Read the model definition and answer for the solid it produces. Units are mm, in the model's axes. A direction names the side the tool comes from. Give positions to 0.01 mm unless a question says otherwise; leave off trailing zeros. Write each loop counter-clockwise with the first axis right and the second up, starting at its lowest first coordinate (ties: lowest second). Pieces come first, ordered by that corner, then holes. Notation, with made-up numbers: M 10.5,31 L 48.5,31 A25 cw 48.5,60 Z; hole C 48.25,78 d6. An arc over 180 degrees is marked long. Put each result on its own line as item: value.
from build123d import *

# Parameters (mm, degrees)
SKETCH1_W           = 40
SKETCH1_H           = 12
SKETCH1_R           = 2
BOSS_EXTRUDE1_DEPTH = 5
SKETCH2_W           = 30.175
SKETCH2_H           = 10
BOSS_EXTRUDE2_DEPTH = 6
SKETCH3_R           = 3.175
CUT_EXTRUDE1_DEPTH  = 17


with BuildPart() as part:
    # Sketch1 → Boss-Extrude1 (new body)
    with BuildSketch(Plane(origin=(0, 0, 0), x_dir=(0, 0, -1), z_dir=(1, 0, 0))):
        Rectangle(SKETCH1_W, SKETCH1_H)
        with Locations((-16, 0)):
            Circle(SKETCH1_R, mode=Mode.SUBTRACT)
        with Locations(Location((16, 0, 0), (0, 0, 180))):
            Circle(SKETCH1_R, mode=Mode.SUBTRACT)
    extrude(amount=BOSS_EXTRUDE1_DEPTH)

    # Sketch2 → Boss-Extrude2 (add, symmetric)
    with BuildSketch(Plane(origin=(0, 0, 0), x_dir=(1, 0, 0), z_dir=(0, 1, 0))):
        with Locations((20.0875, 0)):
            Rectangle(SKETCH2_W, SKETCH2_H)
    extrude(amount=BOSS_EXTRUDE2_DEPTH, both=True)

    # Sketch3 → Cut-Extrude1 (cut, symmetric)
    with BuildSketch(Plane.XY):
        with Locations((35.18, 0)):
            Circle(SKETCH3_R)
    extrude(amount=CUT_EXTRUDE1_DEPTH, both=True, mode=Mode.SUBTRACT)


solid = part.part
(1) Section D-D on z = 8 is taken. Determine the outline of the cut face in (x, y).
Result:
outline: M 0,-6 L 5,-6 L 5,6 L 0,6 Z
(2) Which of the six approach directions +Z, -Z, +X, -X, +Y, -Y give full straight-line access (tool end or side, diameter ignored) to faces 1 (the face through (5, 0, -12)), 2 (the face through (0, 0, 0)), 3 (the face through (5, 0, 13))?
Result:
face 1: -Z, +X, +Y, -Y
face 2: +Z, -Z, -X, +Y, -Y
face 3: +Z, +X, +Y, -Y
(3) Section A-A on y = 0 is taken. Determine the outline of the cut face in (x, z) (3 decimals), and give its area (3 significant figures).
Result:
outline: M 0,-20 L 5,-20 L 5,-18 L 0,-18 Z; M 0,-14 L 5,-14 L 5,-5 L 32.005,-5 L 32.005,5 L 5,5 L 5,14 L 0,14 Z; M 0,18 L 5,18 L 5,20 L 0,20 Z
area: 430 mm²
(4) For a pull along Y with two mould halves and no side action, classify faces 4 (the face through (20, 0, -5)), 5 (the face through (13, -6, 0)), 6 (the face through (32.006, 0.07, 0.07)) as +Y half, -Y half, draft (parallel to the pull), parting line (faces both ways), or undercut.
Result:
face 4: draft
face 5: -Y half
face 6: undercut
(5) Section B-B on z = 16 is taken. Determine the outline of the cut face in (x, y), and give its area (3 significant figures).
Result:
outline: M 0,-6 L 5,-6 L 5,-2 L 0,-2 Z; M 0,2 L 5,2 L 5,6 L 0,6 Z
area: 40.0 mm²
(6) Section C-C on y = -4.25 is taken. Determine the outline of the cut face in (x, z) (3 decimals).
Result:
outline: M 0,-20 L 5,-20 L 5,-5 L 35.175,-5 L 35.175,5 L 5,5 L 5,20 L 0,20 Z
(7) Straight lines are drawn through the part: line 1 along Y through (x, z) = (1, -16); line 2 along Z through (x, y) = (22.5, 4.5); line 3 along X through (y, z) = (-4.75, 6). For each, find the intervals that lie inside material, in ascending order. Write a range as from..to.
Result:
line 1: y = -6..-2, 2..6
line 2: z = -5..5
line 3: x = 0..5
(8) Given pin 1 Ø4 at (x, y) = (13.5, -3) entering from +Z; pin 2 Ø3 at (y, z) = (-1.5, -8) entering from +X; pin 3 Ø1 at (x, y) = (26, -2.5) entering from -Z, each flat-ended and moving along its own axis, determine where each tip first touches the part or whether it passes through.
Result:
pin 1: stops at z = 5
pin 2: stops at x = 5
pin 3: stops at z = -5
